Autodesk Inventor part; units mm, degrees
ref_plane "YZ Plane" through (0, 0, 0) normal (1, 0, 0) x (0, 1, 0)
ref_plane "XZ Plane" through (0, 0, 0) normal (0, 1, 0) x (-1, 0, 0)
ref_plane "XY Plane" through (0, 0, 0) normal (0, 0, 1) x (1, 0, 0)
sketch "Sketch8" plane through (0, 0, 0) normal (0, 1, 0) x (-1, 0, 0)
  circle A0 centre (0, 0) radius 8.509
  dimension "d28" = 17.018
extrude "Extrusion7" add sketch "Sketch8" along normal blind 2.54
sketch "Sketch9" plane through (0, 0, 0) normal (1, 0, 0) x (0, 1, 0)
  line L0 (0, 8.509) -> (2.54, 8.509)
  line L1 (2.54, 8.509) -> (2.54, -8.509)
  line L2 (0, -8.509) -> (2.54, -8.509)
  line L3 (2.54, 8.509) -> (2.54, -8.509)
  line L4 (2.54, -8.509) -> (11.0639, -5.0629)
  line L5 (2.54, 8.509) -> (11.0639, 5.0629)
  arc A0 (11.0639, -5.0629) -> (11.0639, 5.0629) centre (9.017, 0) ccw
  circle A1 centre (9.017, 0) radius 2.667
  line L6 (-3.0224, 0) -> (5.6412, 0) construction
  line L7 (14.478, 5.5398) -> (14.478, 0.9968) construction
  point P0 (0, 0)
  dimension "d31" = 10.922
  dimension "d32" = 5.334
  dimension "d33" = 11.938
extrude "Extrusion8" add sketch "Sketch9" along normal mid plane 6.096
sketch "Sketch10" plane through (0, 2.54, 0) normal (0, 1, 0) x (1, 0, 0)
  arc A0 (3.048, -7.9444) -> (3.048, 7.9444) centre (0, 0) ccw
  circle A1 centre (0, 0) radius 8.509
  circle A2 centre (0, 0) radius 9.0384
  arc A3 (-3.048, 7.9444) -> (-3.048, -7.9444) centre (0, 0) ccw
  point P0 (-3.048, 8.509)
extrude "Extrusion9" cut sketch "Sketch10" along normal blind 12.7
sketch "Sketch11" plane through (0, 0, 0) normal (0, -1, 0) x (1, 0, 0)
  circle A0 centre (0, 0) radius 8.509
  circle A1 centre (0, 0) radius 1.9812
  arc A2 (-6.2682, 1.016) -> (-6.2682, -1.016) centre (0, 0) ccw
  line L0 (-6.2682, 1.016) -> (-4.3273, 1.016)
  line L1 (-6.2682, -1.016) -> (-4.3273, -1.016)
  arc A3 (-1.016, -6.2682) -> (1.016, -6.2682) centre (0, 0) ccw
  line L2 (-1.016, -6.2682) -> (-1.016, -4.3273)
  line L3 (1.016, -6.2682) -> (1.016, -4.3273)
  arc A4 (6.2682, -1.016) -> (6.2682, 1.016) centre (0, 0) ccw
  line L4 (6.2682, -1.016) -> (4.3273, -1.016)
  line L5 (6.2682, 1.016) -> (4.3273, 1.016)
  arc A5 (1.016, 6.2682) -> (-1.016, 6.2682) centre (0, 0) ccw
  line L6 (1.016, 6.2682) -> (1.016, 4.3273)
  line L7 (-1.016, 6.2682) -> (-1.016, 4.3273)
  arc A6 (-1.016, 4.3273) -> (-4.3273, 1.016) centre (0, 0) ccw
  arc A7 (4.3273, 1.016) -> (1.016, 4.3273) centre (0, 0) ccw
  arc A8 (-4.3273, -1.016) -> (-1.016, -4.3273) centre (0, 0) ccw
  arc A9 (1.016, -4.3273) -> (4.3273, -1.016) centre (0, 0) ccw
  dimension "d38" = 3.9624
  dimension "d40" = 12.7
  dimension "d41" = 2.032
  dimension "d42" = 1.016
  dimension "d45" = 360
extrude "Extrusion10" add sketch "Sketch11" along normal blind 15.748 contours L0 A6 L7 A5 L6 A7 L5 A4 L4 A9 L3 A3 L2 A8 L1 A2
sketch "Sketch12" plane through (0, -15.748, 0) normal (0, -1, 0) x (1, 0, 0)
  circle A0 centre (0, 0) radius 1.9812
  arc A1 (1.016, 6.2682) -> (-1.016, 6.2682) centre (0, 0) ccw
  circle A2 centre (0, 0) radius 1.9812
  circle A3 centre (0, 0) radius 3.937
  dimension "d49" = 7.874
extrude "Extrusion11" add sketch "Sketch12" along normal blind 2.032
properties part number "Shock Mount - Bottom"
Read the model definition and answer for the solid it produces. Units are mm, in the model's axes. A direction names the side the tool comes from. Round coordinates to 2 decimals unless told otherwise and drop trailing zeros. Write each loop counter-clockwise with the first axis right and the second up, starting at its lowest first coordinate (ties: lowest second). Pieces come first, ordered by that corner, then holes. Notation, with made-up numbers: (-33, -7.75) - (25, -7.75) arc R20 cw to (25, 10.25) - close; hole circle Ø11 at (-15, -33.75). An arc over 180 degrees is marked (long way). Use a Markdown table: item, result.
(1) The part is cut by section A-A (z = 0). Write down the section's boundary in (x, y).
Reported:
| item | result |
|---|---|
| outline | (-8.51, 0) - (-6.35, 0) - (-6.35, -15.75) - (-3.94, -15.75) - (-3.94, -17.78) - (-1.98, -17.78) - (-1.98, 0) - (1.98, 0) - (1.98, -17.78) - (3.94, -17.78) - (3.94, -15.75) - (6.35, -15.75) - (6.35, 0) - (8.51, 0) - (8.51, 2.54) - (3.05, 2.54) - (3.05, 6.35) - (-3.05, 6.35) - (-3.05, 2.54) - (-8.51, 2.54) - close; (-3.05, 11.68) - (3.05, 11.68) - (3.05, 14.48) - (-3.05, 14.48) - close |
(2) Which of the six approach directions +Z, -Z, +X, -X, +Y, -Y give full straight-line access (tool end or side, diameter ignored) to faces 1 (the cylindrical face through (3.119, -7.764, 3.167)), 2 (the cylindrical face through (-6.35, -7.76, -0.01)), 3 (the flat face through (-1.016, -8, -5)), 4 (the flat face through (5, 2.54, 0))?
Reported:
| item | result |
|---|---|
| face 1 | +Z, +X, -Y |
| face 2 | -X, -Y |
| face 3 | -Z, -X, -Y |
| face 4 | +Z, -Z, +X, +Y |
(3) The part is cut by section D-D (x = 7). Write down the section's boundary in (y, z), then the cut area to 3 significant figures.
Reported:
| item | result |
|---|---|
| outline | (0, -4.84) - (2.54, -4.84) - (2.54, 4.84) - (0, 4.84) - close |
| area | 24.6 mm2 |
(4) Each of these flat-tipped pins is pushed along its axis until it touches: pin 1 Ø2 at (y, z) = (-11, 5.5) entering from -X; pin 2 Ø0.6 at (x, y) = (-5.5, -7.5) entering from +Z; pin 3 Ø1.5 at (x, y) = (6.5, -11.5) entering from -Z; pin 4 Ø2 at (x, z) = (-1, -0.5) entering from -Y. Where does it stop, or does it pass through?
Reported:
| item | result |
|---|---|
| pin 1 | x = -1.02 |
| pin 2 | z = 1.02 |
| pin 3 | z = -1.02 |
| pin 4 | y = -17.78 |
(5) The part is cut by section C-C (y = 0.5). Write down the section's boundary in (x, z).
Reported:
| item | result |
|---|---|
| outline | circle Ø17.02 at (0, 0) |
(6) The part is cut by section B-B (y = -5.5). Write down the section's boundary in (x, z).
Reported:
| item | result |
|---|---|
| outline | (-6.27, -1.02) - (-4.33, -1.02) arc R4.44 ccw to (-1.02, -4.33) - (-1.02, -6.27) arc R6.35 ccw to (1.02, -6.27) - (1.02, -4.33) arc R4.44 ccw to (4.33, -1.02) - (6.27, -1.02) arc R6.35 ccw to (6.27, 1.02) - (4.33, 1.02) arc R4.44 ccw to (1.02, 4.33) - (1.02, 6.27) arc R6.35 ccw to (-1.02, 6.27) - (-1.02, 4.33) arc R4.44 ccw to (-4.33, 1.02) - (-6.27, 1.02) arc R6.35 ccw to start; hole circle Ø3.96 at (0, 0) |
(7) The mould has two halves that part along Y. Classify faces 5 (the flat face through (-2, -17.78, -1)), 6 (the flat face through (-0.04, 6.74, -6.81)), 7 (the flat face through (-5, -8, -1.016)), 8 (the cylindrical face through (-0.04, 11.56, -0.8)): released by +Y, released by -Y, zero draft, split by the parting line, or undercut.
Reported:
| item | result |
|---|---|
| face 5 | released by -Y |
| face 6 | released by +Y |
| face 7 | zero draft |
| face 8 | undercut |
(8) Straight lines are drawn through the part: line 1 along Z through (x, y) = (0, -10); line 2 along Y through (x, z) = (-4.5, -6); line 3 along X through (y, z) = (4.5, -6.25). For each, find the intervals that lie inside material, in ascending order. Write a range as [from, to].
Reported:
| item | result |
|---|---|
| line 1 | [-6.35, -1.98], [1.98, 6.35] |
| line 2 | [0, 2.54] |
| line 3 | [-3.05, 3.05] |
